from build123d import *

# Parameters (mm, degrees)
SKETCH_1_R          = 2
EXTRUDE_1_DEPTH     = 5
SKETCH_2_W          = 15
SKETCH_2_H          = 14
EXTRUDE_2_DEPTH     = 5
CUT_EXTRUDE_1_DEPTH = 0.5
CUT_EXTRUDE_2_DEPTH = 0.5


# Read off the part's stored shape, not the designer's step: 旋转1
with BuildPart() as part:
    # 草图1 → 凸台-拉伸1 (new body)
    with BuildSketch(Plane(origin=(0, 0, 0), x_dir=(0, 0, -1), z_dir=(1, 0, 0))):
        with BuildLine():
            Line((0, 7), (7, 7))
            Line((7, 7), (7, -7))
            Line((7, -7), (0, -7))
            ThreePointArc((0, -7), (-7, 0), (0, 7))
        make_face()
        Circle(SKETCH_1_R, mode=Mode.SUBTRACT)
    extrude_1 = extrude(amount=EXTRUDE_1_DEPTH)

    # 草图2 → 凸台-拉伸2 (add)
    with BuildSketch(Plane(origin=(0, 0, -7), x_dir=(-1, 0, 0), z_dir=(0, 0, -1))):
        with Locations((2.5, 0)):
            Rectangle(SKETCH_2_W, SKETCH_2_H)
    extrude(amount=EXTRUDE_2_DEPTH)

    # 镜向1: 凸台-拉伸1 across plane
    add(extrude_1.mirror(Plane(origin=(-2.5, 0, 0), x_dir=(0, 0, 1), z_dir=(1, 0, 0))))

    # 旋转1 outline → 旋转1 (revolve)
    with BuildSketch(Plane(origin=(-2.5, 0.001459035, -1.77e-07), x_dir=(1, 0, 0), z_dir=(0, -0.9999999926083961, 0.00012158621526376601))):
        with BuildLine():
            Line((0, -11.99939198), (0, -101.999999911))
            add(Edge.make_bspline(
                [(0, -101.999999911), (0.649374565, -102.000631552), (1.36637391, -101.896134883), (2.14664433, -101.640285677), (2.900713445, -101.175064609), (4.050280545, -100.025777019), (4.488587079, -99.403162649), (4.802259983, -98.694270687), (4.967920299, -97.947271844), (5.003923175, -97.131598303), (5.005854013, -97.042976085), (5.00581972, -96.954701862), (5.003854844, -96.866858155), (4.962482411, -95.929533068), (4.746118591, -95.128843425), (4.388787557, -94.446984897), (3.976314487, -93.90027946), (3.539967456, -93.464038525)],
                knots=[7.026698353, 7.026698353, 7.026698353, 7.026698353, 7.026698353, 7.026698353, 7.854954324, 7.854954324, 7.854954324, 7.854954324, 8.516146676, 8.516146676, 8.516146676, 8.516146676, 8.597007798, 8.597007798, 8.597007798, 8.597007798, 9.38398712, 9.38398712, 9.38398712, 9.38398712, 9.38398712, 9.38398712], degree=5, weights=[1, 1, 1.002166416, 1.000644588, 1, 1, 0.998171528, 0.998141501, 1, 1, 0.999999762, 0.999999775, 1, 1, 1.000698327, 1.001864653, 1, 1]))
            ThreePointArc((3.539967456, -93.464038525), (3.091790234, -91.204536808), (5.009475048, -89.928333148))
            Line((5.009475048, -89.928333148), (4.999999963, -11.99939198))
            Line((4.999999963, -11.99939198), (0, -11.99939198))
        make_face()
    revolve(axis=Axis((-2.5, 0.001459035, -1.77e-07), (0, 0.00012158621526376601, 0.9999999926083961)))

    # 草图5 → 切除-拉伸1 (cut)
    with BuildSketch(Plane.ZY):
        with BuildLine():
            Line((-7, 7), (-7, -7))
            Line((-7, -7), (0, -7))
            ThreePointArc((0, -7), (7, 0), (0, 7))
            Line((0, 7), (-7, 7))
        make_face()
    extrude(amount=-CUT_EXTRUDE_1_DEPTH, mode=Mode.SUBTRACT)


with BuildPart() as mirror_2_1:
    # 镜向2: 凸台-拉伸1 across plane
    add(extrude_1.mirror(Plane(origin=(-2.5, 0, 0), x_dir=(0, 0, 1), z_dir=(1, 0, 0))))


with BuildPart() as part_1:
    add(part.part)

    # 镜向2 united with what the copies tou: union 镜向2_1
    add(mirror_2_1.part)

    # 草图6 → 切除-拉伸2 (cut)
    with BuildSketch(Plane(origin=(-5, 0, 0), x_dir=(0, 0, -1), z_dir=(1, 0, 0))):
        with BuildLine():
            Line((0, 7), (7, 7))
            Line((7, 7), (7, -7))
            Line((7, -7), (0, -7))
            ThreePointArc((0, -7), (-7, 0), (0, 7))
        make_face()
    extrude(amount=-CUT_EXTRUDE_2_DEPTH, mode=Mode.SUBTRACT)


solid = part_1.part
Design review of the part built by this model. Coordinates are the model's own, in mm. A direction names the side the tool comes from. Round coordinates to 2 decimals unless told otherwise and drop trailing zeros. Order: outer loops, then holes, each group sorted by start corner. A loop starts at its lowest first (then second) coordinate and runs counter-clockwise, first axis right, second up. Notation, with made-up numbers: M 87,56 L 104,56 A21 cw 104,88 Z; hole C 76.25,45 d3. An arc over 180 degrees is marked long. Answer as CSV lines item,"result". Start each with the question number.
1) The part is to be moulded in two halves that separate along Y. For faces 1 (the face through (-2.4, 7, -7.2)), 2 (the face through (-8, -2, 0)), 3 (the face through (-5.5, -1, -2)), 4 (the face through (-2.4, -7, -7.4)), say which applies: +Y half, -Y half, draft (parallel to the pull), parting line (faces both ways), or undercut.
2) Tool access review of faces 5 (the face through (5, -0.1, -2.4)), 6 (the face through (0.5, -1, -2)): name each direction out of +Z, -Z, +X, -X, +Y, -Y from which nothing blocks a thin tool from reaching the whole face with its end or side.
3) Wall thickness on line 1 along Y through (x, z) = (-6.75, 0); line 2 along X through (y, z) = (-0.5, -73); line 3 along X through (y, z) = (4, -53): over which ranges is each line inside the solid? List them lowest first. Write a range as [from, to].
4) Add section A-A (x = 3.5). Give the boundary of the cut face in (y, z).
5) Add section B-B (y = 1). Give the number of separate pieces and of enclosed holes in the cut face, then the cut area to 3 significant figures.
6) For pin 1 Ø4 at (y, z) = (4, -53.5) entering from -X; pin 2 Ø6 at (x, y) = (-2, 5.5) entering from -Z; pin 3 Ø4.5 at (y, z) = (0, 0) entering from +X; pin 4 Ø6 at (x, y) = (3.5, -2) entering from -Z, all flat-tipped, find the tip position at first contact; note any pin that passes through.
Resolved:
1,face 1,"+Y half"
1,face 2,"undercut"
1,face 3,"draft"
1,face 4,"-Y half"
2,face 5,"+Z, -Z, +X, +Y, -Y"
2,face 6,"+Z, +Y, -Y"
3,line 1,"[-7, -2], [2, 7]"
3,line 2,"[-7.48, 2.48]"
3,line 3,"[-5.5, 0.5]"
4,outline,"M -7,-12 L 7,-12 L 7,0 A7 ccw -7,0 Z; hole C 0,0 d4"
5,separate pieces,"3"
5,enclosed holes,"0"
5,area,"1,020 mm^2"
6,pin 1,"x = -7.09"
6,pin 2,"z = -101.31"
6,pin 3,"x = 5"
6,pin 4,"z = -100.74"
